Geometry: final body of the model. Coordinates: model frame, mm. Face numbers are marked on the shaded views. A direction names the side the tool comes from. Round coordinates to 2 decimals unless told otherwise and drop trailing zeros. Loops run counter-clockwise (first coordinate to the right, second up) from the corner with the lowest first, then second, coordinate; pieces in that order, holes last. Notation, with made-up numbers: (80.25, 59.25) -> (115.25, 59.25) arc R9 ccw to (115.25, 71.25) -> close; hole circle Ø7 at (27, 53). An arc over 180 degrees is marked (long way). Answer in a Markdown table with one row per item.
```python
from build123d import *

# Parameters (mm, degrees)
BOSS_EXTRUDE1_DEPTH = 46.8
SKETCH5_W           = 40
SKETCH5_H           = 15
CUT_EXTRUDE1_DEPTH  = 4
BOSS_EXTRUDE3_DEPTH = 5
SKETCH13_W          = 10
SKETCH13_H          = 2
CUT_EXTRUDE2_DEPTH  = 37


with BuildPart() as part:
    # Sketch1 → Boss-Extrude1 (new body)
    with BuildSketch(Plane(origin=(0, 0, 0), x_dir=(1, 0, 0), z_dir=(0, 1, 0))):
        with BuildLine():
            Line((-82, -20), (82, -20))
            ThreePointArc((82, -20), (85.535533906, -18.535533906), (87, -15))
            Line((87, -15), (87, 5))
            ThreePointArc((87, 5), (82.606601718, 15.606601718), (72, 20))
            Line((72, 20), (-72, 20))
            ThreePointArc((-72, 20), (-82.606601718, 15.606601718), (-87, 5))
            Line((-87, 5), (-87, -15))
            ThreePointArc((-87, -15), (-85.535533906, -18.535533906), (-82, -20))
        make_face()
        with BuildLine():
            Line((-68.08, 16), (68.08, 16))
            add(Edge.make_bspline(
                [(83, 2.5), (83, 16), (68.08, 16)],
                knots=[0, 0, 0, 1.570796327, 1.570796327, 1.570796327], degree=2, weights=[1, 0.707106781, 1]))
            Line((83, 2.5), (83, -16))
            Line((83, -16), (-83, -16))
            Line((-83, -16), (-83, 2.5))
            add(Edge.make_bspline(
                [(-68.08, 16), (-83, 16), (-83, 2.5)],
                knots=[4.71238898, 4.71238898, 4.71238898, 6.283185307, 6.283185307, 6.283185307], degree=2, weights=[1, 0.707106781, 1]))
        make_face(mode=Mode.SUBTRACT)
    extrude(amount=BOSS_EXTRUDE1_DEPTH)

    # Sketch5 → Cut-Extrude1 (cut)
    with BuildSketch(Plane.XY.offset(20)):
        with Locations((-0.5, 7.5)):
            Rectangle(SKETCH5_W, SKETCH5_H)
    extrude(amount=-CUT_EXTRUDE1_DEPTH, mode=Mode.SUBTRACT)

    # Sketch10 → Boss-Extrude3 (add)
    with BuildSketch(Plane(origin=(0, 46.8, 0), x_dir=(1, 0, 0), z_dir=(0, 1, 0))):
        with BuildLine():
            Line((-82, -20), (82, -20))
            ThreePointArc((82, -20), (85.535533906, -18.535533906), (87, -15))
            Line((87, -15), (87, 5))
            ThreePointArc((87, 5), (82.606601718, 15.606601718), (72, 20))
            Line((72, 20), (-72, 20))
            ThreePointArc((-72, 20), (-82.606601718, 15.606601718), (-87, 5))
            Line((-87, 5), (-87, -15))
            ThreePointArc((-87, -15), (-85.535533906, -18.535533906), (-82, -20))
        make_face()
    extrude(amount=BOSS_EXTRUDE3_DEPTH)

    # Sketch13 → Cut-Extrude2 (cut)
    with BuildSketch(Plane.XY.offset(20)):
        with Locations((12.5, 45.8)):
            Rectangle(SKETCH13_W, SKETCH13_H)
    extrude(amount=-CUT_EXTRUDE2_DEPTH, mode=Mode.SUBTRACT)


solid = part.part
```
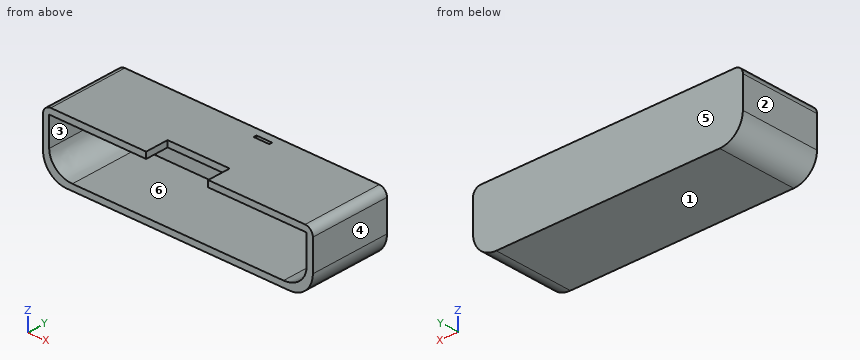
Item 1: First-contact query: P1, Ø3, axis at x = 6, z = -9, coming from the -Y side; P2, Ø2, axis at y = 46, z = 19, coming from the -X side; P3, Ø4.5, axis at x = 8, z = 17.5, coming from the -Y side. Flat tips, straight axial feed; report the tip coordinate or a pass-through.
Ans:
| item | result |
|---|---|
| P1 | y = 46.8 |
| P2 | x = -86 |
| P3 | y = 15 |
Item 2: Mould query, pull axis X, two halves, no side actions, for the marked faces 1, 2, 3 and 4. Classes: released by +X, released by -X, zero draft, split by the parting line, or undercut.
Ans:
| item | result |
|---|---|
| face 1 | zero draft |
| face 2 | released by -X |
| face 3 | undercut |
| face 4 | released by +X |
Item 3: Set-up query: the marked faces 5 and 6. Return all of +Z, -Z, +X, -X, +Y, -Y with unobstructed straight access to the full face (end or side cutting, diameter ignored); none if empty.
Ans:
| item | result |
|---|---|
| face 5 | +Z, -Z, +X, -X, +Y |
| face 6 | -Y |
Item 4: Section query B-B, the plane z = 12. Output: boundary loops of the cut face in (x, y).
Ans:
| item | result |
|---|---|
| outline | (-87, 0) -> (-83, 0) -> (-83, 46.8) -> (83, 46.8) -> (83, 0) -> (87, 0) -> (87, 51.8) -> (-87, 51.8) -> close |
Item 5: Section query A-A, the plane x = 25.5. Output: boundary loops of the cut face in (y, z), and give its area (3 significant figures).
Ans:
| item | result |
|---|---|
| outline | (0, -20) -> (51.8, -20) -> (51.8, 20) -> (0, 20) -> (0, 16) -> (46.8, 16) -> (46.8, -16) -> (0, -16) -> close |
| area | 574 mm2 |
Item 6: Ray query, L1, parallel to X at y = 25.5, z = 9; L2, parallel to Z at x = 16.5, y = 40; L3, parallel to Z at x = 10, y = 4.5. Return the intervals inside material, ascending.
Ans:
| item | result |
|---|---|
| L1 | -87 to -83, 83 to 87 |
| L2 | -20 to -16, 16 to 20 |
| L3 | -20 to -16 |
